from build123d import *

# Parameters (mm, degrees)
SKETCH_1_W          = 57
SKETCH_1_H          = 57
EXTRUDE_3_DEPTH     = 24
SKETCH_3_R          = 28.5
EXTRUDE_4_DEPTH     = 44.8
SKETCH_4_W          = 57
SKETCH_4_H          = 57
EXTRUDE_5_DEPTH     = 10
SKETCH_6_R          = 7
EXTRUDE_6_DEPTH     = 30
SKETCH_7_R          = 2.75
CUT_EXTRUDE_1_DEPTH = 30
SKETCH_8_R          = 2
CUT_EXTRUDE_2_DEPTH = 5


with BuildPart() as part:
    # 草图1 → 凸台-拉伸3 (new body)
    with BuildSketch(Plane(origin=(0, 0, 0), x_dir=(1, 0, 0), z_dir=(0, 1, 0))):
        Rectangle(SKETCH_1_W, SKETCH_1_H)
    extrude(amount=EXTRUDE_3_DEPTH)

    # 草图3 → 凸台-拉伸4 (add)
    with BuildSketch(Plane(origin=(0, 24, 0), x_dir=(1, 0, 0), z_dir=(0, 1, 0))):
        Circle(SKETCH_3_R)
    extrude(amount=EXTRUDE_4_DEPTH)

    # 草图4 → 凸台-拉伸5 (add)
    with BuildSketch(Plane(origin=(0, 68.8, 0), x_dir=(1, 0, 0), z_dir=(0, 1, 0))):
        Rectangle(SKETCH_4_W, SKETCH_4_H)
    extrude(amount=EXTRUDE_5_DEPTH)

    # 草图6 → 凸台-拉伸6 (add)
    with BuildSketch(Plane(origin=(0, 78.8, 0), x_dir=(1, 0, 0), z_dir=(0, 1, 0))):
        Circle(SKETCH_6_R)
    extrude(amount=EXTRUDE_6_DEPTH)

    # 草图7 → 切除-拉伸1 (cut)
    with BuildSketch(Plane(origin=(0, 78.8, 0), x_dir=(1, 0, 0), z_dir=(0, 1, 0))):
        with Locations((23.57, -23.57)):
            Circle(SKETCH_7_R)
        with Locations((-23.57, -23.57)):
            Circle(SKETCH_7_R)
        with Locations((-23.57, 23.57)):
            Circle(SKETCH_7_R)
        with Locations((23.57, 23.57)):
            Circle(SKETCH_7_R)
    extrude(amount=-CUT_EXTRUDE_1_DEPTH, mode=Mode.SUBTRACT)

    # 草图8 → 切除-拉伸2 (cut)
    with BuildSketch(Plane(origin=(0, 0, 0), x_dir=(-1, 0, 0), z_dir=(0, -1, 0))):
        with Locations((23.57, 23.57)):
            Circle(SKETCH_8_R)
        with Locations((-23.57, 23.57)):
            Circle(SKETCH_8_R)
        with Locations((-23.57, -23.57)):
            Circle(SKETCH_8_R)
        with Locations((23.57, -23.57)):
            Circle(SKETCH_8_R)
    extrude(amount=-CUT_EXTRUDE_2_DEPTH, mode=Mode.SUBTRACT)


solid = part.part
For this review, take the finished solid that the model builds, in its own axes (mm). A direction names the side the tool comes from. Coordinates: 2 decimals unless noted, no trailing zeros. Order: outer loops, then holes, each group sorted by start corner. A loop starts at its lowest first (then second) coordinate and runs counter-clockwise, first axis right, second up. Notation, with made-up numbers: (56, 27) - (71, 27) arc R18 ccw to (71, 35) - close; hole circle Ø9 at (43.25, 18). An arc over 180 degrees is marked (long way). Use one line per item in the form item = value.
Q1. Consider section A-A (x = -23.57). Give the boundary of the cut face in (y, z).
Checked values:
outline = (0, -28.5) - (24, -28.5) - (24, -16.02) - (68.8, -16.02) - (68.8, -20.82) - (78.8, -20.82) - (78.8, 20.82) - (68.8, 20.82) - (68.8, 16.02) - (24, 16.02) - (24, 28.5) - (0, 28.5) - (0, 25.57) - (5, 25.57) - (5, 21.57) - (0, 21.57) - (0, -21.57) - (5, -21.57) - (5, -25.57) - (0, -25.57) - close; (68.8, -28.5) - (78.8, -28.5) - (78.8, -26.32) - (68.8, -26.32) - close; (68.8, 26.32) - (78.8, 26.32) - (78.8, 28.5) - (68.8, 28.5) - close
Q2. For faces 1 (the flat face through (-23, 24, 22)), 2 (the flat face through (-24, 5, 24)), 3 (the cylindrical face through (6.466, 93.59, 2.681)), 4 (the flat face through (20.5, 68.8, 22.6)), 5 (the flat face through (-22, 68.8, -21)), list the 3-axis set-ups (+Z, -Z, +X, -X, +Y, -Y) from which the entire face can be reached by the end or side of a thin tool; tool diameter is ignored.
Checked values:
face_1 = +Z, -X
face_2 = -Y
face_3 = +Y
face_4 = +Z, +X
face_5 = -Z, -X
Q3. For P1, Ø8.5, axis at x = -15.5, z = 20.5, coming from the +Y side; P2, Ø8, axis at x = 12, y = 63, coming from the -Z side; P3, Ø4, axis at x = -4, y = 42.5, coming from the -Z side, all flat-tipped, find the tip position at first contact; note any pin that passes through.
Checked values:
P1 = 78.8
P2 = -27.35
P3 = -28.43
Q4. For probe 1 along X at (y, z) = (3.65, -23.57); probe 2 along X at (y, z) = (75.25, 23.57), list the stretches that pass through material, from the lowest coordinate up. Write a range as from..to.
Checked values:
probe_1 = -28.5..-25.57, -21.57..21.57, 25.57..28.5
probe_2 = -28.5..-26.32, -20.82..20.82, 26.32..28.5
Q5. Consider section C-C (x = 16). Give the boundary of the cut face in (y, z).
Checked values:
outline = (0, -28.5) - (24, -28.5) - (24, -23.58) - (68.8, -23.58) - (68.8, -28.5) - (78.8, -28.5) - (78.8, 28.5) - (68.8, 28.5) - (68.8, 23.58) - (24, 23.58) - (24, 28.5) - (0, 28.5) - close
Q6. Draft analysis for pull direction X (two halves, no side actions). For faces 6 (the flat face through (-28.5, 12, 0)), 7 (the flat face through (24, 5, -24)), 8 (the flat face through (22, 24, -23)), state which applies: +X half, -X half, draft (parallel to the pull), parting line (faces both ways), or undercut.
Checked values:
face_6 = -X half
face_7 = undercut
face_8 = draft
Q7. Consider section B-B (z = -23.57). Give the boundary of the cut face in (x, y), then the cut area to 3 significant figures.
Checked values:
outline = (-28.5, 0) - (-25.57, 0) - (-25.57, 5) - (-21.57, 5) - (-21.57, 0) - (21.57, 0) - (21.57, 5) - (25.57, 5) - (25.57, 0) - (28.5, 0) - (28.5, 24) - (16.02, 24) - (16.02, 68.8) - (20.82, 68.8) - (20.82, 78.8) - (-20.82, 78.8) - (-20.82, 68.8) - (-16.02, 68.8) - (-16.02, 24) - (-28.5, 24) - close; (-28.5, 68.8) - (-26.32, 68.8) - (-26.32, 78.8) - (-28.5, 78.8) - close; (26.32, 68.8) - (28.5, 68.8) - (28.5, 78.8) - (26.32, 78.8) - close
area = 3,220 mm2
Q8. Consider section D-D (z = 12). Give the boundary of the cut face in (x, y).
Checked values:
outline = (-28.5, 0) - (28.5, 0) - (28.5, 24) - (25.85, 24) - (25.85, 68.8) - (28.5, 68.8) - (28.5, 78.8) - (-28.5, 78.8) - (-28.5, 68.8) - (-25.85, 68.8) - (-25.85, 24) - (-28.5, 24) - close
